Geometry check sheet. Reference: the model listing, model coordinates, mm. A direction names the side the tool comes from. Give positions to 0.01 mm unless a question says otherwise; leave off trailing zeros. Order: outer loops, then holes, each group sorted by start corner. A loop starts at its lowest first (then second) coordinate and runs counter-clockwise, first axis right, second up. Notation, with made-up numbers: M 32.5,-28 L 71.5,-28 A14 cw 71.5,-5 Z; hole C 52,8 d6. An arc over 180 degrees is marked long. Answer as CSV lines item,"result". Start each with the question number.
Q1. Mould release check, pull along Y, two halves, no side actions. Record for faces 1 (the flat face through (254, 0, -13)), 2 (the cylindrical face through (508.72, -16.46, -1.57)), 3 (the flat face through (515, -7, -3)), 4 (the cylindrical face through (24.002, -10.015, -1.565)): +Y half, -Y half, draft (parallel to the pull), parting line (faces both ways), or undercut.
Q2. Go/stop test with flat-tipped pins: pin 1 (2 mm diameter, centred on x = 415.5, z = -21, fed in from +Y); pin 2 (1 mm diameter, centred on x = 143, y = -16, fed in from -Z) (3 decimals); pin 3 (2 mm diameter, centred on x = 296.5, z = -3.5, fed in from -Y); pin 4 (3 mm diameter, centred on y = -20.5, z = -6, fed in from -X). Record where each tip stops, or that it passes through.
Q3. Thickness scan on line 1 (X direction, y = -12.85, z = -0.9); line 2 (Y direction, x = 15, z = -0.75); line 3 (X direction, y = -14.5, z = -2). Record the ranges inside material, lowest first.
Q4. Section check B-B, the plane x = 44.5. Record the boundary of the cut face in (y, z) (3 decimals).
Q5. Set-up check for faces 5 (the flat face through (0, -7, -3)), 6 (the flat face through (254, -3.175, -15)): record each of +Z, -Z, +X, -X, +Y, -Y from which the full face is reachable in a straight line by a thin tool's end or side.
Q6. Section check A-A, the plane y = -12.85. Record the boundary of the cut face in (x, z) (1 decimal).
Q7. Section check C-C, the plane z = -8.75. Record the boundary of the cut face in (x, y) (3 decimals), then the cut area to 3 significant figures.
Autodesk Inventor part; units mm, degrees
ref_plane "YZ Plane" through (0, 0, 0) normal (1, 0, 0) x (0, 1, 0)
ref_plane "XZ Plane" through (0, 0, 0) normal (0, 1, 0) x (-1, 0, 0)
ref_plane "XY Plane" through (0, 0, 0) normal (0, 0, 1) x (1, 0, 0)
sketch "Boceto1" plane through (0, 0, 0) normal (1, 0, 0) x (0, 1, 0)
  line L0 (0, -0.3) -> (0, -25.4)
  line L1 (-0.3, 0) -> (-25.4, 0)
  arc A0 (0, -0.3) -> (-0.3, 0) centre (-0.3, -0.3) ccw
  line L2 (-25.4, 0) -> (-25.4, -3.175)
  line L3 (0, -25.4) -> (-3.175, -25.4)
  line L4 (-3.175, -25.4) -> (-3.175, -3.475)
  line L5 (-3.475, -3.175) -> (-25.4, -3.175)
  arc A1 (-3.175, -3.475) -> (-3.475, -3.175) centre (-3.475, -3.475) ccw
  point P0 (0, 0)
  dimension "d0" = 25.4
  dimension "d1" = 25.4
  dimension "d2" = 0.3
  dimension "d3" = 3.175
  dimension "d4" = 3.175
  dimension "d5" = 0.3
extrude "Extrusión1" add sketch "Boceto1" along normal blind 515
fillet "Empalme1" radius 2 4 edges at (515, -25.4, -1.5875) (515, -1.5875, -25.4) (0, -25.4, -1.5875) (0, -1.5875, -25.4)
sketch "Boceto3" plane through (0, -0.3, 0) normal (0, 0, 1) x (1, 0, 0)
  line L0 (0, 0) -> (515, 0) construction
  line L1 (257.5, 0) -> (257.5, -25.1) construction
  line L2 (2, -25.1) -> (513, -25.1) construction
  line L3 (257.5, -12.55) -> (500, -12.55) construction
  line L4 (257.5, -12.55) -> (15, -12.55) construction
  circle A0 centre (15, -12.55) radius 9.4375
  circle A1 centre (500, -12.55) radius 9.4375
  dimension "d11" = 242.5
  dimension "d12" = 242.5
  dimension "d13" = 18.875
  dimension "d16" = 18.875
extrude "Extrusión2" cut sketch "Boceto3" against normal up to surface (3.175 mm away)
sketch "Boceto4" plane through (0, -0.3, 0) normal (0, 0, 1) x (1, 0, 0)
  arc A0 (13.9157, -3.175) -> (16.0843, -3.175) centre (15, -12.55) ccw
  line L0 (2, -25.1) -> (513, -25.1) construction
  line L1 (30, -23.1) -> (30, 0) construction
  line L2 (0, 0) -> (515, 0) construction
  line L3 (28, -25.1) -> (2, -25.1) construction
  arc A1 (28, -25.1) -> (30, -23.1) centre (28, -23.1) ccw
  circle A2 centre (500, -12.55) radius 9.4375 construction
  line L4 (515, -23.1) -> (515, -3.175) construction
  line L5 (485, -23.1) -> (485, 0) construction
  line L6 (487, -25.1) -> (513, -25.1) construction
  arc A3 (485, -23.1) -> (487, -25.1) centre (487, -23.1) ccw
  line L7 (485, -23.1) -> (30, -23.1)
  line L8 (28, -25.1) -> (487, -25.1)
  point P0 (0, 0.3)
  point P1 (30, -25.1)
  point P2 (485, -25.1)
  dimension "d20" = 2
  dimension "d23" = 2
extrude "Extrusión3" cut sketch "Boceto4" against normal up to surface (3.175 mm away)
properties part number "angulo_caja_calor" material "Acero inoxidable AISI 304"
Answer block:
1,face 1,"+Y half"
1,face 2,"undercut"
1,face 3,"draft"
1,face 4,"undercut"
2,pin 1,"stops at y = 0"
2,pin 2,"stops at z = -3.175"
2,pin 3,"stops at y = -23.4"
2,pin 4,"passes through"
3,line 1,"x = 0 to 5.56, 24.44 to 490.56, 509.44 to 515"
3,line 2,"y = -25.4 to -22.29, -3.41 to 0"
3,line 3,"x = 0 to 5.71, 24.29 to 490.71, 509.29 to 515"
4,outline,"M -23.4,-3.175 L -3.475,-3.175 A0.3 cw -3.175,-3.475 L -3.175,-25.4 L 0,-25.4 L 0,-0.3 A0.3 ccw -0.3,0 L -23.4,0 Z"
5,face 5,"+Z, -Z, -X, +Y, -Y"
5,face 6,"-Z, +X, -X, -Y"
6,outline,"M 0,-3.2 L 5.6,-3.2 L 5.6,0 L 0,0 Z; M 24.4,-3.2 L 490.6,-3.2 L 490.6,0 L 24.4,0 Z; M 509.4,-3.2 L 515,-3.2 L 515,0 L 509.4,0 Z"
7,outline,"M 0,-3.175 L 515,-3.175 L 515,0 L 0,0 Z"
7,area,"1,640 mm2"
